from build123d import *

# Parameters (mm, degrees)
SKETCH1_W           = 20
SKETCH1_H           = 20
BOSS_EXTRUDE2_DEPTH = 1
SKETCH1_6_W         = 22
SKETCH1_6_H         = 22
SKETCH1_6_W_2       = 20
SKETCH1_6_H_2       = 20
BOSS_EXTRUDE3_DEPTH = 4
SKETCH2_R           = 0.4
BOSS_EXTRUDE4_DEPTH = 0.5
FILLET1_R           = 1.5


with BuildPart() as part:
    # Sketch1 → Boss-Extrude2 (new body)
    with BuildSketch(Plane(origin=(0, 0, 0), x_dir=(1, 0, 0), z_dir=(0, 1, 0))):
        Rectangle(SKETCH1_W, SKETCH1_H)
    extrude(amount=BOSS_EXTRUDE2_DEPTH)

    # Sketch1<6> → Boss-Extrude3 (add)
    with BuildSketch(Plane(origin=(0, 0, 0), x_dir=(1, 0, 0), z_dir=(0, 1, 0))):
        Rectangle(SKETCH1_6_W, SKETCH1_6_H)
        Rectangle(SKETCH1_6_W_2, SKETCH1_6_H_2, mode=Mode.SUBTRACT)
    extrude(amount=BOSS_EXTRUDE3_DEPTH)

    # Sketch2 → Boss-Extrude4 (add)
    with BuildSketch(Plane(origin=(0, 4, 0), x_dir=(1, 0, 0), z_dir=(0, 1, 0))):
        with Locations((0, 10.490155688)):
            Circle(SKETCH2_R)
        with Locations((1, 10.490155688)):
            Circle(SKETCH2_R)
        with Locations((-1, 10.490155688)):
            Circle(SKETCH2_R)
    extrude(amount=BOSS_EXTRUDE4_DEPTH)

    # Fillet1
    fillet1_edges = [part.edges().sort_by_distance(p)[0] for p in [
        (10, 2.5, -10),
        (-10, 2.5, -10),
        (-10, 2.5, 10),
        (10, 2.5, 10),
    ]]
    fillet(fillet1_edges, radius=FILLET1_R)


solid = part.part
Model file for the job. Use its own axes, mm. A direction names the side the tool comes from. Coordinates: 2 decimals unless noted, no trailing zeros. Write each loop counter-clockwise with the first axis right and the second up, starting at its lowest first coordinate (ties: lowest second). Pieces come first, ordered by that corner, then holes. Notation, with made-up numbers: (-12.5, -0.5) - (-1.5, -0.5) arc R17 cw to (-1.5, 21.5) - close; hole circle Ø2 at (4, 52). An arc over 180 degrees is marked (long way). Write each question's results on one line, items separated by ' | '. Start each with the question number.
1) Cut at C-C (z = -6.5). Write the cut outline in (x, y).
2) 3-axis set-ups, long thin cutter, end or side, ignore diameter. For faces 4 (the face through (0, 2, -11)), 5 (the face through (10, 2, 0)): which of +Z, -Z, +X, -X, +Y, -Y reach the whole face in a straight line?
3) Probe line 1 along X through (y, z) = (1.3, 5.25); line 2 along Y through (x, z) = (4.25, -2). List the from-to ranges inside material, lowest first. Write a range as from..to.
4) Cut at A-A (y = 3.25). Write the cut outline in (x, z), then the cut area to 3 significant figures.
5) Mould opens along X. For faces 1 (the face through (-9.55, 2.52, 9.57)), 2 (the face through (0, 0, 0)), 3 (the face through (11, 2, 0)) say: pulls with the +X half, pulls with the -X half, needs draft (parallel to the pull), parting line crosses it, or undercut.
6) Cut at D-D (x = 4.75). Write the cut outline in (y, z), then the cut area to 3 significant figures.
7) Flat gauge pin, fed straight in: P1, Ø6.5, axis at x = 4.5, z = -2.5, coming from the +Y side. Where does the tip first touch, or does it go through?
8) Cut at B-B (x = 1). Write the cut outline in (y, z).
Returned:
1) outline: (-11, 0) - (11, 0) - (11, 4) - (10, 4) - (10, 1) - (-10, 1) - (-10, 4) - (-11, 4) - close
2) face 4: -Z, +X, -X, +Y, -Y | face 5: +Y
3) line 1: -11..-10, 10..11 | line 2: 0..1
4) outline: (-11, -11) - (11, -11) - (11, 11) - (-11, 11) - close; hole (-10, -8.5) arc R1.5 ccw to (-8.5, -10) - (8.5, -10) arc R1.5 ccw to (10, -8.5) - (10, 8.5) arc R1.5 ccw to (8.5, 10) - (-8.5, 10) arc R1.5 ccw to (-10, 8.5) - close | area: 85.9 mm^2
5) face 1: undercut | face 2: needs draft | face 3: pulls with the +X half
6) outline: (0, -11) - (4, -11) - (4, -10) - (1, -10) - (1, 10) - (4, 10) - (4, 11) - (0, 11) - close | area: 28.0 mm^2
7) P1: y = 1
8) outline: (0, -11) - (4, -11) - (4, -10.89) - (4.5, -10.89) - (4.5, -10.09) - (4, -10.09) - (4, -10) - (1, -10) - (1, 10) - (4, 10) - (4, 11) - (0, 11) - close
